Read the model definition and answer for the solid it produces. Units are mm, in the model's axes. A direction names the side the tool comes from. Round coordinates to 2 decimals unless told otherwise and drop trailing zeros. Write each loop counter-clockwise with the first axis right and the second up, starting at its lowest first coordinate (ties: lowest second). Pieces come first, ordered by that corner, then holes. Notation, with made-up numbers: (23, 27.5) -> (40, 27.5) arc R21 cw to (40, 39.5) -> close; hole circle Ø2 at (37, -31). An arc over 180 degrees is marked (long way). Return JSON: item names as keys, results as strings.
from build123d import *

# Parameters (mm, degrees)
BOSS_EXTRUDE1_DEPTH = 30
GUSSET1_THICKNESS   = 3
GUSSET2_THICKNESS   = 3
BOSS_EXTRUDE2_DEPTH = 3
BOSS_EXTRUDE3_DEPTH = 3
BOSS_EXTRUDE4_DEPTH = 3
BOSS_EXTRUDE5_DEPTH = 3
CUT_EXTRUDE1_DEPTH  = 58.879184514
CUT_EXTRUDE2_DEPTH  = 13


with BuildPart() as part:
    # Sketch2 → Boss-Extrude1 (new body)
    with BuildSketch(Plane(origin=(0, 0, 0), x_dir=(0, 0, -1), z_dir=(1, 0, 0))):
        Polygon((0, 35), (0, 0), (35, 0), (35, 4), (4, 4), (4, 35), align=None)
    extrude(amount=BOSS_EXTRUDE1_DEPTH)



with BuildPart() as body_2:
    # Gusset1: a gusset: a plate 3.0 thick in the corner of two members, its outline drawn in place
    gusset1_outline = Wire([Line((27, 4, -4), (27, 29, -4)), Line((27, 29, -4), (27, 4, -29)), Line((27, 4, -29), (27, 4, -4))])
    add(extrude(Face(gusset1_outline), amount=GUSSET1_THICKNESS, dir=(1, 0, 0)))


with BuildPart() as body_3:
    # Gusset2: a gusset: a plate 3.0 thick in the corner of two members, its outline drawn in place
    gusset2_outline = Wire([Line((3, 4, -4), (3, 4, -29)), Line((3, 4, -29), (3, 29, -4)), Line((3, 29, -4), (3, 4, -4))])
    add(extrude(Face(gusset2_outline), amount=GUSSET2_THICKNESS, dir=(-1, 0, 0)))


with BuildPart() as part_1:
    add(part.part)

    add(body_2.part)  # Boss-Extrude2 merges body 2
    # Sketch7 → Boss-Extrude2 (add)
    with BuildSketch(Plane(origin=(30, 0, 0), x_dir=(0, 0, -1), z_dir=(1, 0, 0))):
        Polygon((4, 35), (7, 35), (7, 26), (4, 29), align=None)
    extrude(amount=-BOSS_EXTRUDE2_DEPTH)


    add(body_3.part)  # Boss-Extrude3 merges body 3
    # Sketch8 → Boss-Extrude3 (add)
    with BuildSketch(Plane.ZY):
        Polygon((-4, 35), (-7, 35), (-7, 26), (-4, 29), align=None)
    extrude(amount=-BOSS_EXTRUDE3_DEPTH)

    # Sketch9 → Boss-Extrude4 (add)
    with BuildSketch(Plane.ZY):
        Polygon((-35, 4), (-35, 7), (-26, 7), (-29, 4), align=None)
    extrude(amount=-BOSS_EXTRUDE4_DEPTH)

    # Sketch10 → Boss-Extrude5 (add)
    with BuildSketch(Plane(origin=(30, 0, 0), x_dir=(0, 0, -1), z_dir=(1, 0, 0))):
        Polygon((35, 4), (35, 7), (26, 7), (29, 4), align=None)
    extrude(amount=-BOSS_EXTRUDE5_DEPTH)

    # Sketch11 → Cut-Extrude1 (cut, through all)
    with BuildSketch(Plane.XY):
        with BuildLine():
            Line((12, 15), (12, 25))
            ThreePointArc((12, 25), (15, 28), (18, 25))
            Line((18, 25), (18, 15))
            ThreePointArc((18, 15), (15, 12), (12, 15))
        make_face()
    extrude(amount=-CUT_EXTRUDE1_DEPTH, mode=Mode.SUBTRACT)

    # Sketch12 → Cut-Extrude2 (cut)
    with BuildSketch(Plane.XZ):
        with BuildLine():
            Line((12, -22.5), (12, -12.5))
            ThreePointArc((12, -12.5), (15, -9.5), (18, -12.5))
            Line((18, -12.5), (18, -22.5))
            ThreePointArc((18, -22.5), (15, -25.5), (12, -22.5))
        make_face()
    extrude(amount=-CUT_EXTRUDE2_DEPTH, mode=Mode.SUBTRACT)


solid = part_1.part
Item 1: Section C-C (z = -19) is taken. Give the vertices of the cut face in (x, y).
Worked answers:
{"outline": "(0, 0) -> (12, 0) -> (12, 4) -> (3, 4) -> (3, 14) -> (0, 14) -> close; (18, 0) -> (30, 0) -> (30, 14) -> (27, 14) -> (27, 4) -> (18, 4) -> close"}
Item 2: Section A-A (x = 15) is taken. Give the vertices of the cut face in (y, z), then the cut area to 3 significant figures.
Worked answers:
{"outline": "(0, -35) -> (4, -35) -> (4, -25.5) -> (0, -25.5) -> close; (0, -9.5) -> (4, -9.5) -> (4, -4) -> (12, -4) -> (12, 0) -> (0, 0) -> close; (28, -4) -> (35, -4) -> (35, 0) -> (28, 0) -> close", "area": "136 mm2"}
Item 3: For a pull along Z with two mould halves and no side action, classify faces 4 (the flat face through (15, 35, -3)), 5 (the flat face through (12, 2, -18)), 6 (the flat face through (9, 19, -4)) as released by +Z, released by -Z, zero draft, split by the parting line, or undercut.
Worked answers:
{"face 4": "zero draft", "face 5": "undercut", "face 6": "released by -Z"}
Item 4: Straight lines are drawn through the part: L1, parallel to Y at x = 26, z = -15.5; L2, parallel to Z at x = 10.75, y = 12.5; L3, parallel to X at y = 13, z = -5. For each, find the intervals that lie inside material, in ascending order. Write a range as [from, to].
Worked answers:
{"L1": "y = [0, 4]", "L2": "z = [-4, 0]", "L3": "x = [0, 3], [27, 30]"}
Item 5: A tool of negligible diameter and unlimited length cuts with its end or side. For faces 1 (the flat face through (1, 7, -31)), 2 (the flat face through (9, 4, -20)), 3 (the flat face through (18, 2, -17)), from which of +Z, -Z, +X, -X, +Y, -Y can it reach the whole face along a straight path? Write none if from no direction.
Worked answers:
{"face 1": "-Z, +X, -X, +Y", "face 2": "-Z, +Y", "face 3": "+Y, -Y"}
Item 6: Section D-D (x = 19) is taken. Give the vertices of the cut face in (y, z).
Worked answers:
{"outline": "(0, -35) -> (4, -35) -> (4, -4) -> (35, -4) -> (35, 0) -> (0, 0) -> close"}
Item 7: Flat-ended cylindrical pins translate along their axes: pin 1 (0.9 mm diameter, centred on x = 28.5, y = 31, fed in from -Z); pin 2 (1 mm diameter, centred on x = 12, z = -23, fed in from +Y); pin 3 (1.5 mm diameter, centred on x = 29, z = -31.5, fed in from +Y). Find the tip coordinate at first contact, or state that the pin passes through.
Worked answers:
{"pin 1": "stops at z = -7", "pin 2": "stops at y = 4", "pin 3": "stops at y = 7"}
Item 8: Section B-B (y = 16.5) is taken. Give the vertices of the cut face in (x, z), then the cut area to 3 significant figures.
Worked answers:
{"outline": "(0, -16.5) -> (3, -16.5) -> (3, -4) -> (12, -4) -> (12, 0) -> (0, 0) -> close; (18, -4) -> (27, -4) -> (27, -16.5) -> (30, -16.5) -> (30, 0) -> (18, 0) -> close", "area": "171 mm2"}
